```python
from build123d import *

# Parameters (mm, degrees)
F0_W     = 31.75
F0_H     = 31.75
F0_W_2   = 6.35
F0_H_2   = 6.35
F0_R     = 1.5875
F1_DEPTH = 25.4
F2_DEPTH = 3.175


# Not quite as in the source:
# - a length typed as a fraction of an inch, garbled in the dataset ("3 / 203.2 mm" for 3/8 in), is restored


with BuildPart() as f1:
    # F0 (on Front) → F1 (new body)
    with BuildSketch(Plane.XZ):
        with Locations((-5.7344107546, 14.0581134118)):
            Rectangle(F0_W, F0_H)
        with Locations((-12.0844107546, 7.7081134118)):
            Rectangle(F0_W_2, F0_H_2, mode=Mode.SUBTRACT)
        with Locations((-12.0844107546, 14.0581134118)):
            Circle(F0_R, mode=Mode.SUBTRACT)
        with Locations((-5.7344107546, 7.7081134118)):
            Circle(F0_R, mode=Mode.SUBTRACT)
        with Locations((0.6155892454, 7.7081134118)):
            Rectangle(F0_W_2, F0_H_2, mode=Mode.SUBTRACT)
        with Locations((-5.7344107546, 14.0581134118)):
            Circle(F0_R, mode=Mode.SUBTRACT)
        with Locations((0.6155892454, 14.0581134118)):
            Circle(F0_R, mode=Mode.SUBTRACT)
        with Locations((-12.0844107546, 20.4081134118)):
            Rectangle(F0_W_2, F0_H_2, mode=Mode.SUBTRACT)
        with Locations((-5.7344107546, 20.4081134118)):
            Circle(F0_R, mode=Mode.SUBTRACT)
        with Locations((0.6155892454, 20.4081134118)):
            Circle(F0_R, mode=Mode.SUBTRACT)
    extrude(amount=F1_DEPTH)

    # F0 (on Front) → F2 (join)
    with BuildSketch(Plane.XZ):
        with Locations((-5.7344107546, 14.0581134118)):
            Rectangle(F0_W, F0_H)
        with Locations((-12.0844107546, 7.7081134118)):
            Rectangle(F0_W_2, F0_H_2, mode=Mode.SUBTRACT)
        with Locations((-12.0844107546, 14.0581134118)):
            Circle(F0_R, mode=Mode.SUBTRACT)
        with Locations((-5.7344107546, 7.7081134118)):
            Circle(F0_R, mode=Mode.SUBTRACT)
        with Locations((0.6155892454, 7.7081134118)):
            Rectangle(F0_W_2, F0_H_2, mode=Mode.SUBTRACT)
        with Locations((-5.7344107546, 14.0581134118)):
            Circle(F0_R, mode=Mode.SUBTRACT)
        with Locations((0.6155892454, 14.0581134118)):
            Circle(F0_R, mode=Mode.SUBTRACT)
        with Locations((-12.0844107546, 20.4081134118)):
            Rectangle(F0_W_2, F0_H_2, mode=Mode.SUBTRACT)
        with Locations((-5.7344107546, 20.4081134118)):
            Circle(F0_R, mode=Mode.SUBTRACT)
        with Locations((0.6155892454, 20.4081134118)):
            Circle(F0_R, mode=Mode.SUBTRACT)
        with Locations((-12.0844107546, 7.7081134118)):
            Rectangle(F0_W_2, F0_H_2)
        with Locations((-5.7344107546, 7.7081134118)):
            Circle(F0_R)
        with Locations((0.6155892454, 7.7081134118)):
            Rectangle(F0_W_2, F0_H_2)
        with Locations((0.6155892454, 14.0581134118)):
            Circle(F0_R)
        with Locations((-5.7344107546, 14.0581134118)):
            Circle(F0_R)
        with Locations((-12.0844107546, 14.0581134118)):
            Circle(F0_R)
        with Locations((-12.0844107546, 20.4081134118)):
            Rectangle(F0_W_2, F0_H_2)
        with Locations((-5.7344107546, 20.4081134118)):
            Circle(F0_R)
        with Locations((0.6155892454, 20.4081134118)):
            Circle(F0_R)
    extrude(amount=F2_DEPTH)


solid = f1.part
```
Geometry check sheet. Reference: the model listing, model coordinates, mm. A direction names the side the tool comes from. Coordinates: 2 decimals unless noted, no trailing zeros. Order: outer loops, then holes, each group sorted by start corner. A loop starts at its lowest first (then second) coordinate and runs counter-clockwise, first axis right, second up. Notation, with made-up numbers: M -34.75,33.5 L 24.25,33.5 A21 cw 24.25,55.5 Z; hole C 17,76 d4. An arc over 180 degrees is marked long. One line per question, with ' | ' between items. Start each with the question number.
Item 1: Set-up check for faces 5 (the flat face through (-6, 0, 14)), 6 (the flat face through (1, -14, 4.533)): record each of +Z, -Z, +X, -X, +Y, -Y from which the full face is reachable in a straight line by a thin tool's end or side.
Item 2: Draft check along X on faces 1 (the flat face through (10.141, -13, 14)), 2 (the flat face through (3.791, -14, 8)), 3 (the flat face through (-6, -13, -1.817)), 4 (the flat face through (-2.559, -14, 8)). Enter one of: pulls with the +X half, pulls with the -X half, needs draft (parallel to the pull), parting line crosses it, or undercut.
Item 3: Material ranges on L1, parallel to X at y = -23.75, z = 5; L2, parallel to Z at x = -15, y = -17; L3, parallel to Z at x = 3, y = -16.25, recorded low to high. Write a range as [from, to].
Item 4: Cross-section at C-C on x = 1. Enter the section's corners in (y, z) (3 decimals).
Item 5: Cross-section at D-D on z = 10. Enter the section's corners in (x, y) (3 decimals), then the cut area to 3 significant figures.
Item 6: Cross-section at A-A on y = -23. State how many separate pieces and enclosed holes the cut face has, then the cut area to 3 significant figures.
Item 7: Gauge pin test, flat ends, axial feed: pin 1 (10 mm diameter, centred on x = 0.5, z = 21.5, fed in from +Y); pin 2 (2.5 mm diameter, centred on x = -5.73, z = 7.71, fed in from -Y) (3 decimals). Record the tip position at first contact, or that the pin passes through.
Item 8: Cross-section at B-B on z = 18. Enter the section's corners in (x, y) (3 decimals), then the cut area to 3 significant figures.
Findings:
1) face 5: +Z, -Z, +X, -X, +Y | face 6: -Y
2) face 1: pulls with the +X half | face 2: undercut | face 3: needs draft | face 4: undercut
3) L1: x = [-21.61, -15.26], [-8.91, -2.56], [3.79, 10.14] | L2: z = [-1.82, 4.53], [10.88, 17.23], [23.58, 29.93] | L3: z = [-1.82, 4.53], [10.88, 29.93]
4) outline: M -25.4,-1.817 L 0,-1.817 L 0,29.933 L -25.4,29.933 L -25.4,21.948 L -3.175,21.948 L -3.175,18.868 L -25.4,18.868 L -25.4,15.598 L -3.175,15.598 L -3.175,12.518 L -25.4,12.518 L -25.4,10.883 L -3.175,10.883 L -3.175,4.533 L -25.4,4.533 Z
5) outline: M -21.609,-25.4 L -15.259,-25.4 L -15.259,-3.175 L -8.909,-3.175 L -8.909,-25.4 L -2.559,-25.4 L -2.559,-3.175 L 3.791,-3.175 L 3.791,-25.4 L 10.141,-25.4 L 10.141,0 L -21.609,0 Z | area: 524 mm²
6) separate pieces: 1 | enclosed holes: 9 | area: 840 mm²
7) pin 1: stops at y = 0 | pin 2: stops at y = -3.175
8) outline: M -21.609,-25.4 L -15.259,-25.4 L -15.259,-3.175 L -8.909,-3.175 L -8.909,-25.4 L 10.141,-25.4 L 10.141,0 L -21.609,0 Z | area: 665 mm²
